Read the model definition and answer for the solid it produces. Units are mm, in the model's axes. Give positions to 0.01 mm unless a question says otherwise; leave off trailing zeros. Write each loop counter-clockwise with the first axis right and the second up, starting at its lowest first coordinate (ties: lowest second). Pieces come first, ordered by that corner, then holes. Notation, with made-up numbers: (64.25, 49) -> (80.25, 49) arc R23 ccw to (80.25, 60) -> close; hole circle Ø3 at (88.5, 32.25). An arc over 180 degrees is marked (long way). Write item = value, one per line.
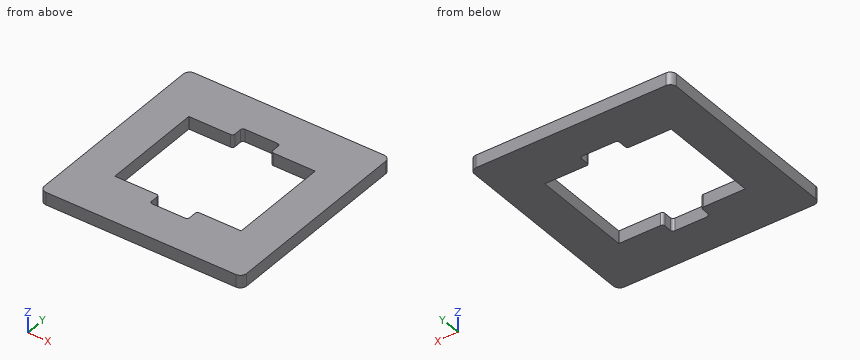
from build123d import *

# Parameters (mm, degrees)
MAINBODYS_W     = 16
MAINBODYS_H     = 16
MAIN_BODY_DEPTH = 1
MIDCUTS_W       = 10
MIDCUTS_H       = 8
MID_CUT_DEPTH   = 12.357816692
GROUNDCUTS_W    = 3
GROUNDCUTS_H    = 1
GROUNDCUT_DEPTH = 12.357816692
OUTER_FILLETS_R = 0.5
GCF_R           = 0.2


with BuildPart() as part:
    # MainBodyS → MAIN BODY (new body)
    with BuildSketch(Plane.XY):
        Rectangle(MAINBODYS_W, MAINBODYS_H)
    extrude(amount=-MAIN_BODY_DEPTH)

    # MidCutS → MID CUT (cut, through all)
    with BuildSketch(Plane.XY):
        Rectangle(MIDCUTS_W, MIDCUTS_H)
    extrude(amount=-MID_CUT_DEPTH, mode=Mode.SUBTRACT)

    # GroundCutS → GroundCut (cut, through all)
    with BuildSketch(Plane.XY):
        with Locations((0, 4.5)):
            Rectangle(GROUNDCUTS_W, GROUNDCUTS_H)
    groundcut = extrude(amount=-GROUNDCUT_DEPTH, mode=Mode.SUBTRACT)

    # GCVM: GroundCut across plane
    add(groundcut.mirror(Plane.ZX), mode=Mode.SUBTRACT)

    # OUTER FILLETS
    outer_fillets_edges = [part.edges().sort_by_distance(p)[0] for p in [
        (8, -8, -0.5),
        (-8, -8, -0.5),
        (-8, 8, -0.5),
        (8, 8, -0.5),
    ]]
    fillet(outer_fillets_edges, radius=OUTER_FILLETS_R)

    # GCF
    gcf_edges = [part.edges().sort_by_distance(p)[0] for p in [
        (1.5, 5, -0.5),
        (1.5, 4, -0.5),
        (-1.5, 4, -0.5),
        (-1.5, 5, -0.5),
        (1.5, -4, -0.5),
        (1.5, -5, -0.5),
        (-1.5, -5, -0.5),
        (-1.5, -4, -0.5),
    ]]
    fillet(gcf_edges, radius=GCF_R)


solid = part.part
(1) The part is cut by section C-C on z = -0.5. Determine the outline of the cut face in (x, y), plus the area to 3 significant figures.
Checks:
outline = (-8, -7.5) arc R0.5 ccw to (-7.5, -8) -> (7.5, -8) arc R0.5 ccw to (8, -7.5) -> (8, 7.5) arc R0.5 ccw to (7.5, 8) -> (-7.5, 8) arc R0.5 ccw to (-8, 7.5) -> close; hole (-5, -4) -> (-1.7, -4) arc R0.2 cw to (-1.5, -4.2) -> (-1.5, -4.8) arc R0.2 ccw to (-1.3, -5) -> (1.3, -5) arc R0.2 ccw to (1.5, -4.8) -> (1.5, -4.2) arc R0.2 cw to (1.7, -4) -> (5, -4) -> (5, 4) -> (1.7, 4) arc R0.2 cw to (1.5, 4.2) -> (1.5, 4.8) arc R0.2 ccw to (1.3, 5) -> (-1.3, 5) arc R0.2 ccw to (-1.5, 4.8) -> (-1.5, 4.2) arc R0.2 cw to (-1.7, 4) -> (-5, 4) -> close
area = 170 mm²
(2) The part is cut by section A-A on x = -0.25. Determine the outline of the cut face in (y, z).
Checks:
outline = (-8, -1) -> (-5, -1) -> (-5, 0) -> (-8, 0) -> close; (5, -1) -> (8, -1) -> (8, 0) -> (5, 0) -> close
(3) Consider L1, parallel to X at y = 3.75, z = -0.35; L2, parallel to Y at x = 4.25, z = -0.35. Determine where each line is inside the solid, lowest interval first.
Checks:
L1 = -8 to -5, 5 to 8
L2 = -8 to -4, 4 to 8
